```python
from build123d import *

# Parameters (mm, degrees)
SKETCH1_R           = 18
SKETCH1_R_2         = 10.75
BOSS_EXTRUDE1_DEPTH = 14
BOSS_EXTRUDE2_DEPTH = 6
BOSS_EXTRUDE3_START = 24
SKETCH6_R           = 10
BOSS_EXTRUDE3_DEPTH = 24
SKETCH7_R           = 3.25
CUT_EXTRUDE1_DEPTH  = 64.812224534


with BuildPart() as part:
    # Sketch1 → Boss-Extrude1 (new body)
    with BuildSketch(Plane(origin=(0, 0, 0), x_dir=(1, 0, 0), z_dir=(0, 1, 0))):
        with Locations(Location((0, 0, 0), (0, 0, 270))):
            Circle(SKETCH1_R)
        with Locations(Location((0, 0, 0), (0, 0, 270))):
            Circle(SKETCH1_R_2, mode=Mode.SUBTRACT)
    extrude(amount=BOSS_EXTRUDE1_DEPTH)

    # Sketch1_4 → Boss-Extrude2 (add)
    with BuildSketch(Plane(origin=(0, 0, 0), x_dir=(1, 0, 0), z_dir=(0, 1, 0))):
        with BuildLine():
            ThreePointArc((40.105263158, -9.775881906), (48, 0), (40.105263158, 9.775881906))
            Line((40.105263158, 9.775881906), (3.789473684, 17.59658743))
            ThreePointArc((3.789473684, 17.59658743), (14.003758894, 11.309055524), (18, 0))
            ThreePointArc((18, 0), (14.003758894, -11.309055524), (3.789473684, -17.59658743))
            Line((3.789473684, -17.59658743), (40.105263158, -9.775881906))
        make_face()
    extrude(amount=BOSS_EXTRUDE2_DEPTH)

    # Sketch6 → Boss-Extrude3 (add)
    with BuildSketch(Plane.XZ.offset(BOSS_EXTRUDE3_START)):
        with Locations(Location((38, 0, 0), (0, 0, 270))):
            Circle(SKETCH6_R)
    extrude(amount=-BOSS_EXTRUDE3_DEPTH)

    # Sketch7 → Cut-Extrude1 (cut, through all)
    with BuildSketch(Plane.XZ.offset(24)):
        with Locations(Location((38, 0, 0), (0, 0, 270))):
            Circle(SKETCH7_R)
    extrude(amount=-CUT_EXTRUDE1_DEPTH, mode=Mode.SUBTRACT)


solid = part.part
```
Model file for the job. Use its own axes, mm. Round coordinates to 2 decimals unless told otherwise and drop trailing zeros. Order: outer loops, then holes, each group sorted by start corner. A loop starts at its lowest first (then second) coordinate and runs counter-clockwise, first axis right, second up. Notation, with made-up numbers: (65.5, 63.5) -> (72.5, 63.5) arc R5 cw to (72.5, 68.5) -> close; hole circle Ø6 at (-0.75, 12). An arc over 180 degrees is marked (long way). Use one line per item in the form item = value.
Item 1: Cut at C-C, the plane z = 8.5. Write the cut outline in (x, y), and give its area (3 significant figures).
Returned:
outline = (-15.87, 0) -> (-6.58, 0) -> (-6.58, 14) -> (-15.87, 14) -> close; (6.58, 0) -> (32.73, 0) -> (32.73, -24) -> (43.27, -24) -> (43.27, 6) -> (15.87, 6) -> (15.87, 14) -> (6.58, 14) -> close
area = 677 mm^2
Item 2: Drill centre lines: line 1 (X direction, y = 7.5, z = 0); line 2 (X direction, y = -8, z = 0); line 3 (Y direction, x = 42, z = -3). Where is each one in solid material? Low to high.
Returned:
line_1 = -18 to -10.75, 10.75 to 18
line_2 = 28 to 34.75, 41.25 to 48
line_3 = -24 to 6
Item 3: Cut at D-D, the plane y = 2.5. Write the cut outline in (x, z), and give its area (3 significant figures).
Returned:
outline = (3.79, -17.6) -> (40.11, -9.78) arc R10 ccw to (40.11, 9.78) -> (3.79, 17.6) arc R18 ccw (long way) to start; hole circle Ø21.5 at (0, 0); hole circle Ø6.5 at (38, 0)
area = 1,360 mm^2
Item 4: Flat gauge pins, fed straight in: pin 1 Ø7.5 at (x, z) = (38, 0) entering from +Y; pin 2 Ø8 at (x, z) = (-9.5, -3) entering from -Y; pin 3 Ø2 at (x, y) = (35.5, -12) entering from -Z. Where does each tip first touch, or does it go through?
Returned:
pin_1 = 6
pin_2 = 0
pin_3 = -9.89
Item 5: Pull direction Z, two halves, no side cores. Call faces 1 (the face through (-17.572, 8.458, -3.902)), 2 (the face through (7.27, 6.9, -7.92)), 3 (the face through (11, 0, 0)): released by +Z, released by -Z, zero draft, split by the parting line, or undercut.
Returned:
face_1 = split by the parting line
face_2 = undercut
face_3 = zero draft
Item 6: Cut at A-A, the plane z = 0. Write the cut outline in (x, y).
Returned:
outline = (-18, 0) -> (-10.75, 0) -> (-10.75, 14) -> (-18, 14) -> close; (10.75, 0) -> (28, 0) -> (28, -24) -> (34.75, -24) -> (34.75, 6) -> (18, 6) -> (18, 14) -> (10.75, 14) -> close; (41.25, -24) -> (48, -24) -> (48, 6) -> (41.25, 6) -> close
Item 7: Cut at B-B, the plane x = -6. Write the cut outline in (y, z).
Returned:
outline = (0, -16.97) -> (14, -16.97) -> (14, -8.92) -> (0, -8.92) -> close; (0, 8.92) -> (14, 8.92) -> (14, 16.97) -> (0, 16.97) -> close
